Autodesk Inventor part; units mm, degrees
ref_plane "YZ Plane" through (0, 0, 0) normal (1, 0, 0) x (0, 1, 0)
ref_plane "XZ Plane" through (0, 0, 0) normal (0, 1, 0) x (-1, 0, 0)
ref_plane "XY Plane" through (0, 0, 0) normal (0, 0, 1) x (1, 0, 0)
sketch "Эскиз1" plane through (0, 0, 0) normal (0, 0, 1) x (1, 0, 0)
  circle A0 centre (0, 0) radius 1.5
  dimension "d0" = 3
extrude "Выдавливание1" add sketch "Эскиз1" along normal blind 41.25
sketch "Эскиз2" plane through (0, 0, 41.25) normal (0, 0, 1) x (1, 0, 0)
  line L0 (-1.5, -1) -> (1.5, -1)
  line L1 (1.5, -1) -> (1.5, 1)
  line L2 (1.5, 1) -> (-1.5, 1)
  line L3 (-1.5, 1) -> (-1.5, -1)
  line L4 (-1.5, -1) -> (1.5, 1) construction
  line L5 (1.5, -1) -> (-1.5, 1) construction
  circle A0 centre (0, 0) radius 1.5
  point P0 (-1.118, 1)
  point P1 (1.118, 1)
  dimension "d3" = 2
extrude "Выдавливание2" cut sketch "Эскиз2" against normal blind 8 contours A0 L2
sketch "Эскиз3" plane through (0, 0, 0) normal (0, 0, -1) x (-1, 0, 0)
  arc A0 (1.118, 1) -> (-1.118, 1) centre (0, 0) ccw
  line L0 (-1.118, 1) -> (1.118, 1)
extrude "Выдавливание3" cut sketch "Эскиз3" against normal blind 5
equation "\"Радиус_гибки\" = Толщина"
equation "\"Ширина_просечки\" = Толщина"
equation "\"Глубина_просечки\" = 0.5 * Толщина"
equation "\"Размер_просечки\" = 4 * Толщина"
equation "\"Мин_остаток\" = 2 * Толщина"
equation "\"Радиус_перехода\" = Радиус_гибки"
equation "\"Радиус_Якоби\" = Толщина"
equation "\"Размер_зазора\" = Толщина"
properties part number "Ось 3мм задняя"
For this review, take the finished solid that the model builds, in its own axes (mm). A direction names the side the tool comes from. Give positions to 0.01 mm unless a question says otherwise; leave off trailing zeros. Order: outer loops, then holes, each group sorted by start corner. A loop starts at its lowest first (then second) coordinate and runs counter-clockwise, first axis right, second up.
1) For faces 1 (the face through (0, 0, 41.25)), 2 (the face through (0, 1, 2)), 3 (the face through (0, 1, 37)), list the 3-axis set-ups (+Z, -Z, +X, -X, +Y, -Y) from which the entire face can be reached by the end or side of a thin tool; tool diameter is ignored.
2) Take a section at A-A (x = 0). Give the boundary of the cut face in (y, z).
3) Insertion check: pin 1 (0.5 mm diameter, centred on x = -0.5, y = 1, fed in from -Z); pin 2 (1 mm diameter, centred on y = -1, z = 7, fed in from +X); pin 3 (1.1 mm diameter, centred on x = 0.5, z = 2, fed in from +Y). Each pin has a flat end and moves straight along its axis. Give the tip position at first contact, or say it passes through.
4) Take a section at C-C (y = -0.4). Give the boundary of the cut face in (x, z).
5) Take a section at B-B (z = 8). Give the boundary of the cut face in (x, y).
6) Take a section at D-D (z = 37). Give the boundary of the cut face in (x, y).
7) Wall thickness on line 1 (X direction, y = 1, z = 10.5); line 2 (X direction, y = -0.1, z = 3); line 3 (Y direction, x = 0.8, z = 7.5): over which ranges is each line inside the solid? List them lowest first.
Derived:
1. face 1: +Z, +X, -X, +Y, -Y
1. face 2: -Z, +X, -X, +Y
1. face 3: +Z, +X, -X, +Y
2. outline: (-1.5, 0) - (1, 0) - (1, 5) - (1.5, 5) - (1.5, 33.25) - (1, 33.25) - (1, 41.25) - (-1.5, 41.25) - close
3. pin 1: stops at z = 0
3. pin 2: stops at x = 1.41
3. pin 3: stops at y = 1
4. outline: (-1.45, 0) - (1.45, 0) - (1.45, 41.25) - (-1.45, 41.25) - close
5. outline: circle Ø3 at (0, 0)
6. outline: (-1.12, 1) arc R1.5 ccw (long way) to (1.12, 1) - close
7. line 1: x = -1.12 to 1.12
7. line 2: x = -1.5 to 1.5
7. line 3: y = -1.27 to 1.27
